Input: dimensioned drawing with shaded views. Units: mm. Origin: part minimum x, y, z. Round coordinates to 2 decimals unless told otherwise and drop trailing zeros. Write each loop counter-clockwise with the first axis right and the second up, starting at its lowest first coordinate (ties: lowest second). Pieces come first, ordered by that corner, then holes. Notation, with made-up numbers: M 57,13.5 L 97,13.5 A16 ccw 97,35.5 Z; hole C 88.25,34 d11. An arc over 180 degrees is marked long. Answer in a Markdown table with one row per item. Add a question column.
Item 1: Contact query for flat-ended pins moving along their axis: pin 1 (6.5 mm diameter, centred on x = 28.5, z = 16, fed in from +Y); pin 2 (5 mm diameter, centred on x = 16, z = 3.5, fed in from -Y); pin 3 (2 mm diameter, centred on x = 9.5, y = 2.5, fed in from +Z) (3 decimals). Output: stop coordinate, or through.
Item 2: Cut plane A-A on z = 16. Return loops of the section in (x, y), and give its area (3 significant figures).
Item 3: Mould query, pull axis X, two halves, no side actions, for the marked faces 1, 2 and 3. Classes: released by +X, released by -X, zero draft, split by the parting line, or undercut.
Item 4: Cut plane D-D on z = 3.5. Return loops of the section in (x, y).
Item 5: Cut plane C-C on x = 3.5. Return loops of the section in (y, z).
Item 6: Cut plane B-B on y = 0.55. Return loops of the section in (x, z), and give its area (3 significant figures).
Item 7: Material intervals for probe 1 along X at (y, z) = (1.5, 16); probe 2 along Z at (x, y) = (15, 2.55), sorted ascending.
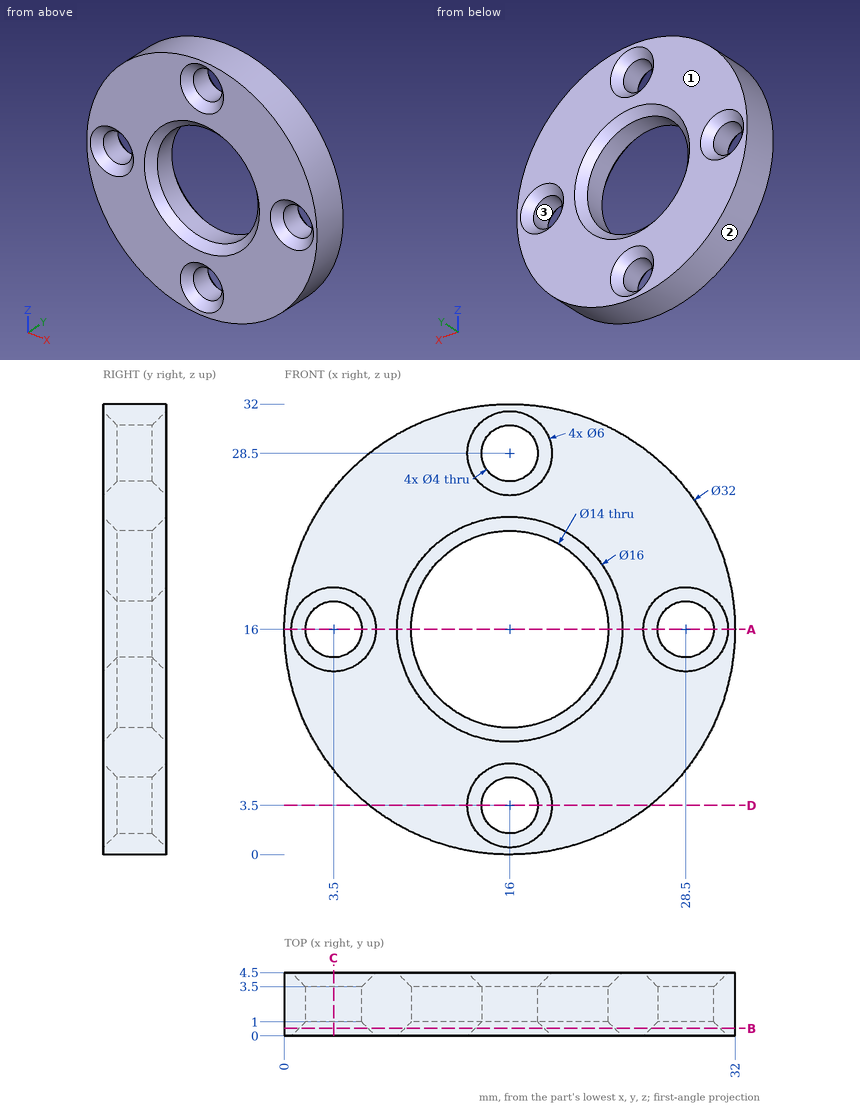
Results below:
| question | item | result |
|---|---|---|
| 1 | pin 1 | y = 4.5 |
| 1 | pin 2 | y = 0.5 |
| 1 | pin 3 | z = 31.025 |
| 2 | outline | M 0,0 L 0.5,0 L 1.5,1 L 1.5,3.5 L 0.5,4.5 L 0,4.5 Z; M 5.5,1 L 6.5,0 L 8,0 L 9,1 L 9,3.5 L 8,4.5 L 6.5,4.5 L 5.5,3.5 Z; M 23,1 L 24,0 L 25.5,0 L 26.5,1 L 26.5,3.5 L 25.5,4.5 L 24,4.5 L 23,3.5 Z; M 30.5,1 L 31.5,0 L 32,0 L 32,4.5 L 31.5,4.5 L 30.5,3.5 Z |
| 2 | area | 39.0 mm2 |
| 3 | face 1 | zero draft |
| 3 | face 2 | split by the parting line |
| 3 | face 3 | undercut |
| 4 | outline | M 6.01,0 L 13,0 L 14,1 L 14,3.5 L 13,4.5 L 6.01,4.5 Z; M 18,1 L 19,0 L 25.99,0 L 25.99,4.5 L 19,4.5 L 18,3.5 Z |
| 5 | outline | M 0,6.01 L 4.5,6.01 L 4.5,13 L 3.5,14 L 1,14 L 0,13 Z; M 0,19 L 1,18 L 3.5,18 L 4.5,19 L 4.5,25.99 L 0,25.99 Z |
| 6 | outline | C 16,16 d32; hole C 3.5,16 d4.9; hole C 16,16 d14.9; hole C 16,3.5 d4.9; hole C 16,28.5 d4.9; hole C 28.5,16 d4.9 |
| 6 | area | 554 mm2 |
| 7 | probe 1 | 0 to 1.5, 5.5 to 9, 23 to 26.5, 30.5 to 32 |
| 7 | probe 2 | 0.03 to 1.77, 5.23 to 9.07, 22.93 to 26.77, 30.23 to 31.97 |
